Verification items for the finished model (mm, model axes). A direction names the side the tool comes from. Round coordinates to 2 decimals unless told otherwise and drop trailing zeros. Order: outer loops, then holes, each group sorted by start corner. A loop starts at its lowest first (then second) coordinate and runs counter-clockwise, first axis right, second up. Notation, with made-up numbers: (25.5, 68.25) -> (68.5, 68.25) arc R30 cw to (68.5, 104.25) -> close; hole circle Ø6 at (47.25, 2.25). An arc over 180 degrees is marked (long way). Put each result on its own line as item: value.
```python
from build123d import *

# Parameters (mm, degrees)
F0_R     = 60.626412
F2_DEPTH = 70.271613
F3_DEPTH = 18.127655


with BuildPart() as f2:
    # F0 (on Top) → F2 (new body)
    with BuildSketch(Plane.XY):
        Circle(F0_R)
    extrude(amount=F2_DEPTH)

    # F1 (on face) → F3 (join)
    with BuildSketch(Plane.XY):
        Polygon((-20.55445, 52.941081), (-54.206494, 16.938108), (-47.039942, -31.819606), (-4.451355, -56.616507), (41.489194, -38.780024), (56.187533, 8.258608), (28.575514, 49.07834), align=None)
    extrude(amount=-F3_DEPTH)


solid = f2.part
```
Item 1: Sectioned sample at C-C, the plane y = 0. Record the boundary of the cut face in (x, z).
Geometry check:
outline: (-60.63, 0) -> (-51.72, 0) -> (-51.72, -18.13) -> (53.61, -18.13) -> (53.61, 0) -> (60.63, 0) -> (60.63, 70.27) -> (-60.63, 70.27) -> close
Item 2: Material ranges on line 1 along Z through (x, y) = (50, -26.5); line 2 along X through (y, z) = (30.5, 21.5); line 3 along Y through (x, z) = (37, -11), recorded low to high.
Geometry check:
line 1: 0 to 70.27
line 2: -52.4 to 52.4
line 3: -40.52 to 36.62
Item 3: Sectioned sample at A-A, the plane x = 22.5. Record the boundary of the cut face in (y, z).
Geometry check:
outline: (-56.3, 0) -> (-46.15, 0) -> (-46.15, -18.13) -> (49.56, -18.13) -> (49.56, 0) -> (56.3, 0) -> (56.3, 70.27) -> (-56.3, 70.27) -> close
Item 4: Sectioned sample at B-B, the plane z = -3. Record the boundary of the cut face in (x, y), then the cut area to 3 significant figures.
Geometry check:
outline: (-54.21, 16.94) -> (-47.04, -31.82) -> (-4.45, -56.62) -> (41.49, -38.78) -> (56.19, 8.26) -> (28.58, 49.08) -> (-20.55, 52.94) -> close
area: 8,830 mm2
Item 5: Depth check by flat-ended pin: pin 1 Ø4 at (y, z) = (46.5, 51) entering from -X; pin 2 Ø4 at (y, z) = (-32.5, 0) entering from +X; pin 3 Ø5 at (x, z) = (21, 48) entering from -Y. Enter the tip coordinate at first touch or a pass-through.
Geometry check:
pin 1: x = -41.17
pin 2: x = 52.4
pin 3: y = -57.73
Item 6: Sectioned sample at D-D, the plane z = 51.5. Record the boundary of the cut face in (x, y), then the cut area to 3 significant figures.
Geometry check:
outline: circle Ø121.25 at (0, 0)
area: 11,500 mm2
Item 7: Tool access check on faces 1 (the face through (18.2, -47.82, -8.94)), 2 (the face through (42.575, 28.383, -8.937)), 3 (the face through (-50.673, -7.099, -8.937)). Record the directions out of +Z, -Z, +X, -X, +Y, -Y that give a thin tool (end or side, any length) a straight path to the whole face; none if there is none.
Geometry check:
face 1: -Z, +X, -Y
face 2: -Z, +X, +Y
face 3: -Z, -X, -Y
